```python
from build123d import *

# Parameters (mm, degrees)
F1_DEPTH = 25.4
F2_R     = 22.86
F3_T     = 1.27


# Not quite as in the source:
# - a shell that OpenCascade refuses in one call is made with other operations: the cavity is built on its own and cut out


with BuildPart() as f1:
    # F0 (on Top) → F1 (new body)
    with BuildSketch(Plane.XY):
        with BuildLine():
            add(Edge.make_bspline(
                [(0, 43.18), (12.6277618203, 28.5479942033), (38.1078160952, 0.5540033901), (12.7566059893, -29.6560009835), (0, -43.18)],
                knots=[0, 0, 0, 0, 0.5, 1, 1, 1, 1], degree=3))
            add(Edge.make_bspline(
                [(0, 43.18), (-12.6384950786, 28.547848961), (-38.0970572555, 0.5541481006), (-12.7673904104, -29.6561451622), (0, -43.18)],
                knots=[0, 0, 0, 0, 0.5, 1, 1, 1, 1], degree=3))
        make_face()
    extrude(amount=F1_DEPTH)

    # F2
    f2_edges = [f1.edges().sort_by_distance(p)[0] for p in [
        (25.400061, -0.050271, 0),
        (-25.400061, -0.050358, 0),
    ]]
    fillet(f2_edges, radius=F2_R)

    # F3: shell of thickness 1.27, made by hand


with BuildPart() as f3_core1:
    # F3_t2: copy of F1
    add(f1.part)

    # the walls: a layer under each face that stays
    f3_faces = [f3_core1.faces().sort_by_distance(p)[0] for p in [
        (25.4, 0, 24.1299999999),
        (-25.4, 0, 24.1299999999),
        (18.704477423, -0.0148216465, 6.6955389821),
        (-18.704477436, -0.0148275323, 6.6955389821),
        (-1.3114e-06, -0.2233707907, 0),
    ]]
    thicken(f3_faces, amount=-F3_T, mode=Mode.SUBTRACT)


with BuildPart() as f1_1:
    add(f1.part)

    # what is left inside the walls is the cavity
    f3_cavity = [f3_core1.part.solids().sort_by_distance(p)[0] for p in [
        (-2e-06, -13.805023, 25.3873),
    ]]
    add(f3_cavity, mode=Mode.SUBTRACT)


solid = f1_1.part
```
Could you check a few things on this model? Use its own coordinates, in mm. Coordinates: 2 decimals unless noted, no trailing zeros. Return JSON: item names as keys, results as strings.
(1) We'd pull the mould along X, two halves only. Please class faces 1 (the flat face through (0, 0, 1.27)), 2 (the flat face through (0, 0, 0)): +X half, -X half, draft (parallel to the pull), parting line (faces both ways), or undercut.
Numbers:
{"face 1": "undercut", "face 2": "draft"}
(2) I'm going to push flat-ended pins straight in: pin 1 (6 mm diameter, centred on y = 18, z = 15.5, fed in from +X); pin 2 (4 mm diameter, centred on x = 1.5, y = 30.5, fed in from +Z); pin 3 (10 mm diameter, centred on y = 23.5, z = 11, fed in from +X). Where does each tip first touch, or does it pass through?
Numbers:
{"pin 1": "stops at x = 20.24", "pin 2": "stops at z = 10.53", "pin 3": "stops at x = 16.64"}
(3) I need wall thicknesses on L1, parallel to Y at x = 18, z = 14; L2, parallel to X at y = 33, z = 15.5; L3, parallel to X at y = -11.5, z = 19. Which ranges of each line are inside material? Lowest first, please.
Numbers:
{"L1": "y = -17.76 to -14.89, 14.48 to 17.3", "L2": "x = -7.14 to -5.38, 5.37 to 7.13", "L3": "x = -22.69 to -21.3, 21.3 to 22.69"}
